For this review, use the dimensioned drawing (mm, ordinates from the lowest corner) and the shaded views. Coordinates: 2 decimals unless noted, no trailing zeros. Loops run counter-clockwise (first coordinate to the right, second up) from the corner with the lowest first, then second, coordinate; pieces in that order, holes last. Notation, with made-up numbers: M 40,68.5 L 46,68.5 A22 ccw 46,99.5 Z; hole C 22.5,0.25 d1. An arc over 180 degrees is marked long. Use CSV: the item, a comma, the result in double quotes. Start each with the question number.
1. Draft analysis for pull direction X (two halves, no side actions). For the marked faces 1 and 2, state which applies: +X half, -X half, draft (parallel to the pull), parting line (faces both ways), or undercut.
2. Add section D-D, the plane z = 64. State how many separate pieces and enclosed holes the cut face has, then the cut area to 3 significant figures.
3. Add section C-C, the plane y = 3.05. Write out the cut boundary in (x, z) (1 decimal), then the cut area to 3 significant figures.
4. Clearance check with flat-ended pins moving along their axes: P1, Ø1.9, axis at x = 64, z = 8, coming from the +Y side; P2, Ø3, axis at x = 8, z = 8, coming from the -Y side. State where each tip first meets the part, or that it passes through.
5. Add section A-A, the plane z = 36. Write out the cut boundary in (x, y).
6. For L1, parallel to Z at x = 36, y = 4.8; L2, parallel to Z at x = 8, y = 2.8; L3, parallel to Z at x = 64, y = 3.2, list the stretches that pass through material, from the lowest coordinate up.
7. Add section B-B, the plane x = 36. Write out the cut boundary in (y, z), then the cut area to 3 significant figures.
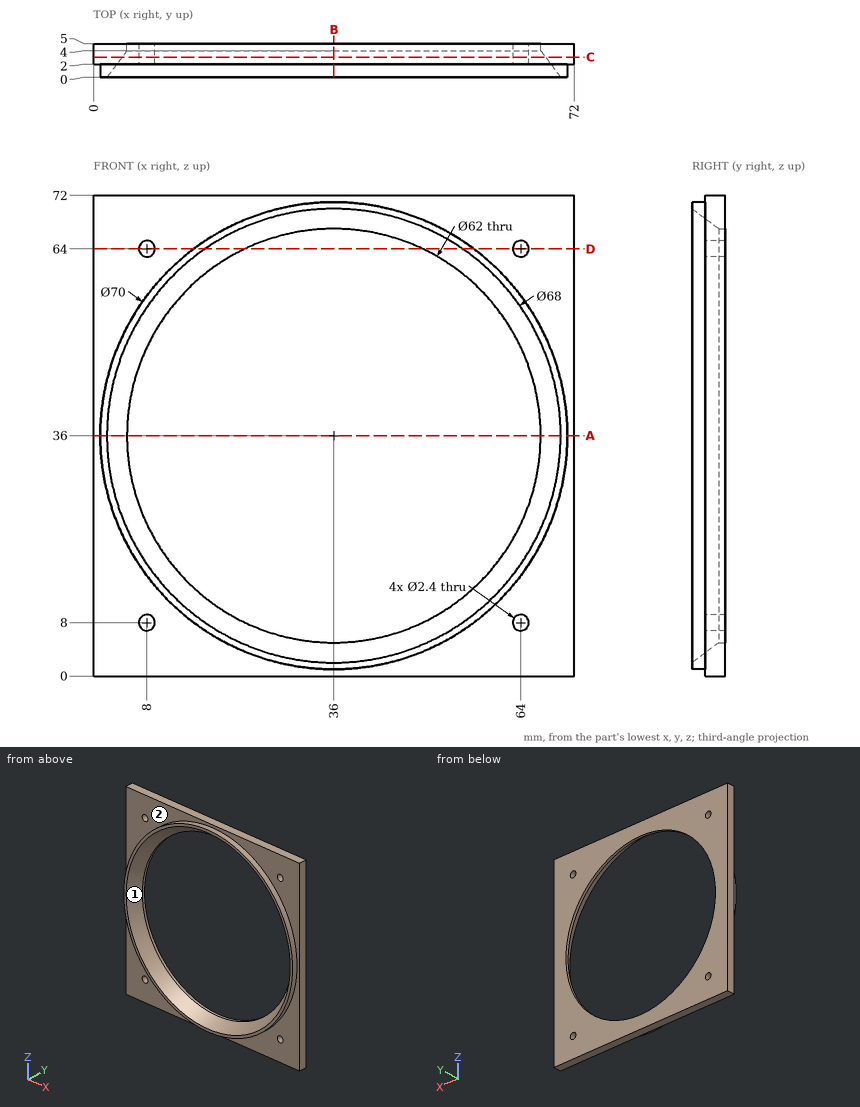
Computed:
1,face 1,"undercut"
1,face 2,"draft"
2,separate pieces,"4"
2,enclosed holes,"0"
2,area,"128 mm^2"
3,outline,"M 0,0 L 72,0 L 72,72 L 0,72 Z; hole C 36,36 d63.4; hole C 8,8 d2.4; hole C 8,64 d2.4; hole C 64,8 d2.4; hole C 64,64 d2.4"
3,area,"2,010 mm^2"
4,P1,"passes through"
4,P2,"stops at y = 2"
5,outline,"M 0,2 L 1,2 L 1,0 L 2,0 L 5,4 L 5,5 L 0,5 Z; M 67,4 L 70,0 L 71,0 L 71,2 L 72,2 L 72,5 L 67,5 Z"
6,L1,"z = 0 to 5, 67 to 72"
6,L2,"z = 0 to 6.8, 9.2 to 20.72, 51.28 to 62.8, 65.2 to 72"
6,L3,"z = 0 to 6.8, 9.2 to 21.35, 50.65 to 62.8, 65.2 to 72"
7,outline,"M 0,1 L 2,1 L 2,0 L 5,0 L 5,5 L 4,5 L 0,2 Z; M 0,70 L 4,67 L 5,67 L 5,72 L 2,72 L 2,71 L 0,71 Z"
7,area,"34.0 mm^2"
